Geometry: final body of the model. Coordinates: model frame, mm. A direction names the side the tool comes from. Coordinates: 2 decimals unless noted, no trailing zeros. Loops run counter-clockwise (first coordinate to the right, second up) from the corner with the lowest first, then second, coordinate; pieces in that order, holes last. Notation, with made-up numbers: (15, -28) -> (63, -28) arc R29 ccw to (63, 6) -> close; hole circle Ø6 at (22.25, 68.25). An arc over 180 degrees is marked (long way). One line per item, written item: value. Start each with the question number.
from build123d import *

# Parameters (mm, degrees)
BOSS_EXTRUDE1_DEPTH       = 4
SKETCH2_W                 = 51
SKETCH2_H                 = 4
BOSS_EXTRUDE2_DEPTH       = 16
BOSS_EXTRUDE3_DEPTH       = 15
SKETCH4_W                 = 51
SKETCH4_H                 = 4
BOSS_EXTRUDE4_DEPTH       = 25
BOSS_EXTRUDE5_DEPTH       = 4
SKETCH6_R                 = 6.5
CUT_EXTRUDE1_DEPTH        = 138.431688125
SKETCH7_R                 = 2.5
CUT_EXTRUDE2_DEPTH        = 127.55618871
CUT_EXTRUDE7_DEPTH        = 10
M3X0_5_TAPPED_HOLE1_D     = 2.6
M3X0_5_TAPPED_HOLE1_DEPTH = 9
M3X0_5_TAPPED_HOLE1_TIP   = 0.781118805
FILLET1_R                 = 5


with BuildPart() as part:
    # Sketch1 → Boss-Extrude1 (new body)
    with BuildSketch(Plane.XY):
        with BuildLine():
            Line((0, 0), (-98.17, 0))
            ThreePointArc((-98.17, 0), (-116.17, 18), (-98.17, 36))
            Line((-98.17, 36), (0, 36))
            Line((0, 36), (0, 0))
        make_face()
    extrude(amount=BOSS_EXTRUDE1_DEPTH)

    # Sketch2 → Boss-Extrude2 (add)
    with BuildSketch(Plane.XY.offset(4)):
        with Locations((-25.5, 2)):
            Rectangle(SKETCH2_W, SKETCH2_H)
    extrude(amount=BOSS_EXTRUDE2_DEPTH)

    # Sketch3 → Boss-Extrude3 (add)
    with BuildSketch(Plane.XY.offset(20)):
        with BuildLine():
            Line((-51, 1.1e-08), (-51, 4.000000011))
            Line((-51, 4.000000011), (-41, 4.000000011))
            Line((-41, 4.000000011), (-41, 18.000000011))
            Line((-41, 18.000000011), (-21, 18.000000011))
            Line((-21, 18.000000011), (-21, 36.000000011))
            Line((-21, 36.000000011), (39.000002857, 35.999993821))
            ThreePointArc((39.000002857, 35.999993821), (56.999993821, 17.999998572), (39, 6.179e-06))
            Line((39, 6.179e-06), (-51, 1.1e-08))
        make_face()
    extrude(amount=BOSS_EXTRUDE3_DEPTH)

    # Sketch4 → Boss-Extrude4 (add)
    with BuildSketch(Plane.XY.offset(35)):
        with Locations((-25.5, 2)):
            Rectangle(SKETCH4_W, SKETCH4_H)
    extrude(amount=BOSS_EXTRUDE4_DEPTH)

    # Sketch5 → Boss-Extrude5 (add)
    with BuildSketch(Plane.XY.offset(60)):
        with BuildLine():
            Line((0, 0), (-98.17, 0))
            ThreePointArc((-98.17, 0), (-116.17, 18), (-98.17, 36))
            Line((-98.17, 36), (0, 36))
            Line((0, 36), (0, 0))
        make_face()
    extrude(amount=BOSS_EXTRUDE5_DEPTH)

    # Sketch6 → Cut-Extrude1 (cut, through all)
    with BuildSketch(Plane.XY.offset(64)):
        with Locations((-98.17, 18)):
            Circle(SKETCH6_R)
    extrude(amount=-CUT_EXTRUDE1_DEPTH, mode=Mode.SUBTRACT)

    # Sketch7 → Cut-Extrude2 (cut, through all)
    with BuildSketch(Plane.XY.offset(35)):
        with Locations((39, 18)):
            Circle(SKETCH7_R)
    extrude(amount=-CUT_EXTRUDE2_DEPTH, mode=Mode.SUBTRACT)

    # Sketch8 → Cut-Extrude7 (cut)
    with BuildSketch(Plane.XY.offset(35)):
        with BuildLine():
            Line((8.498741262, 4.973372122), (8.498741262, 0))
            Line((8.498741262, 0), (39, 6.179e-06))
            ThreePointArc((39, 6.179e-06), (30.025855334, 2.408885262), (23.448763614, 8.972408358))
            ThreePointArc((23.448763614, 8.972408358), (14.431387141, 12.738878418), (8.498741262, 4.973372122))
        make_face()
    extrude(amount=-CUT_EXTRUDE7_DEPTH, mode=Mode.SUBTRACT)

    # M3x0.5 Tapped Hole1
    with Locations(Plane.XY.offset(35)):
        with Locations((39, 32), (25, 18), (39, 4), (53, 18)):
            Hole(M3X0_5_TAPPED_HOLE1_D / 2, depth=M3X0_5_TAPPED_HOLE1_DEPTH)
            with Locations((0, 0, -(M3X0_5_TAPPED_HOLE1_DEPTH + M3X0_5_TAPPED_HOLE1_TIP / 2))):  # 118° drill point
                Cone(0, M3X0_5_TAPPED_HOLE1_D / 2, M3X0_5_TAPPED_HOLE1_TIP, mode=Mode.SUBTRACT)

    # Fillet1
    fillet1_edges = [part.edges().sort_by_distance(p)[0] for p in [
        (-51, 2, 4),
        (-51, 2, 60),
    ]]
    fillet(fillet1_edges, radius=FILLET1_R)


solid = part.part
1. Line query: L1, parallel to Z at x = -0.5, y = 7; L2, parallel to Z at x = -52, y = 34.5; L3, parallel to X at y = 3, z = 28. Output: solid intervals per line, ascending. Write a range as [from, to].
2. Section B-B on x = -100. Return the cut outline in (y, z), plus the area to 3 significant figures.
3. Pin query (flat end, axial travel): pin 1 Ø2 at (y, z) = (1.5, 43) entering from -X; pin 2 Ø4 at (x, y) = (25.5, 8) entering from +Z; pin 3 Ø4 at (x, y) = (39, 32) entering from -Z; pin 4 Ø6 at (y, z) = (16, 8.5) entering from +X. Return the tip coordinate at first contact, or that it passes through.
4. Section D-D on z = 12. Return the cut outline in (x, y).
5. Set-up query: faces 5 (the face through (-52, 2, 6)), 6 (the face through (17, 5, 25)), 7 (the face through (0, 11.4, 60.2)). Return all of +Z, -Z, +X, -X, +Y, -Y with unobstructed straight access to the full face (end or side cutting, diameter ignored); none if empty.
6. Section A-A on z = 28.5. Return the cut outline in (x, y).
7. Section C-C on y = 28. Return the cut outline in (x, z).
8. Draft query along Y for faces 1 (the face through (41.385, 18.751, 27.605)), 2 (the face through (-50, 36, 62)), 3 (the face through (-91.97, 19.95, 62.03)), 4 (the face through (-51, 2, 32)). Return one class per face: released by +Y, released by -Y, zero draft, split by the parting line, or undercut.
Checks:
1. L1: [0, 4], [20, 35], [60, 64]
1. L2: [0, 4], [60, 64]
1. L3: [-51, 8.5], [29.07, 38.17], [39.83, 48.95]
2. outline: (0.09, 0) -> (11.76, 0) -> (11.76, 4) -> (0.09, 4) -> close; (0.09, 60) -> (11.76, 60) -> (11.76, 64) -> (0.09, 64) -> close; (24.24, 0) -> (35.91, 0) -> (35.91, 4) -> (24.24, 4) -> close; (24.24, 60) -> (35.91, 60) -> (35.91, 64) -> (24.24, 64) -> close
2. area: 187 mm²
3. pin 1: x = -51
3. pin 2: z = 35
3. pin 3: z = 20
3. pin 4: through
4. outline: (-51, 0) -> (0, 0) -> (0, 4) -> (-51, 4) -> close
5. face 5: -X, +Y, -Y
5. face 6: +Z, -Y
5. face 7: +Z, +X, +Y, -Y
6. outline: (-51, 0) -> (8.5, 0) -> (8.5, 4.97) arc R8 cw to (23.45, 8.97) arc R18 ccw to (39, 0) arc R18 ccw to (39, 36) -> (-21, 36) -> (-21, 18) -> (-41, 18) -> (-41, 4) -> (-51, 4) -> close; hole circle Ø2.6 at (25, 18); hole circle Ø5 at (39, 18); hole circle Ø2.6 at (39, 4); hole circle Ø2.6 at (39, 32); hole circle Ø2.6 at (53, 18)
7. outline: (-113.14, 0) -> (0, 0) -> (0, 4) -> (-113.14, 4) -> close; (-113.14, 60) -> (0, 60) -> (0, 64) -> (-113.14, 64) -> close; (-21, 20) -> (53.97, 20) -> (53.97, 35) -> (-21, 35) -> close
8. face 1: undercut
8. face 2: released by +Y
8. face 3: undercut
8. face 4: zero draft
